The listing builds one solid part. Answer for the finished solid, in the listing's coordinates (mm). Face numbers are marked on the shaded views. A direction names the side the tool comes from. Round coordinates to 2 decimals unless told otherwise and drop trailing zeros. Write each loop counter-clockwise with the first axis right and the second up, starting at its lowest first coordinate (ties: lowest second). Pieces come first, ordered by that corner, then holes. Notation, with made-up numbers: M 32,-36.5 L 73,-36.5 A20 cw 73,2.5 Z; hole C -37,29 d1. An arc over 180 degrees is marked long. One line per item, written item: value. Start each with the question number.
(1) Given P1, Ø5, axis at x = -8.5, z = 8.5, coming from the +Y side; P2, Ø6, axis at x = 38, z = 12.5, coming from the -Y side; P3, Ø1.5, axis at y = 4.5, z = 11.5, coming from the +X side, each flat-ended and moving along its own axis, determine where each tip first touches the part or whether it passes through.
(2) For the marked faces 4 and 5, determine the directions among +Z, -Z, +X, -X, +Y, -Y from which every point of the face is accessible in a straight line to the end or side of a thin tool.
(3) Section D-D (x = 49.5) is taken. Determine the outline of the cut face in (y, z), plus the area to 3 significant figures.
(4) Consider probe 1 along Z at (x, y) = (-42.5, 13.5); probe 2 along Y at (x, z) = (0, 7) (3 decimals); probe 3 along X at (y, z) = (-3, 8). Determine where each line is inside the solid, lowest interval first.
(5) For a pull along Y with two mould halves and no side action, classify the marked faces 1, 2 and 3 as released by +Y, released by -Y, zero draft, split by the parting line, or undercut.
(6) Section A-A (x = 0) is taken. Determine the outline of the cut face in (y, z) (3 decimals).
(7) Section B-B (z = 7.5) is taken. State how many separate pieces and enclosed holes the cut face has, plus the area to 3 significant figures.
(8) Section C-C (x = -42.5) is taken. Determine the outline of the cut face in (y, z), plus the area to 4 significant figures.
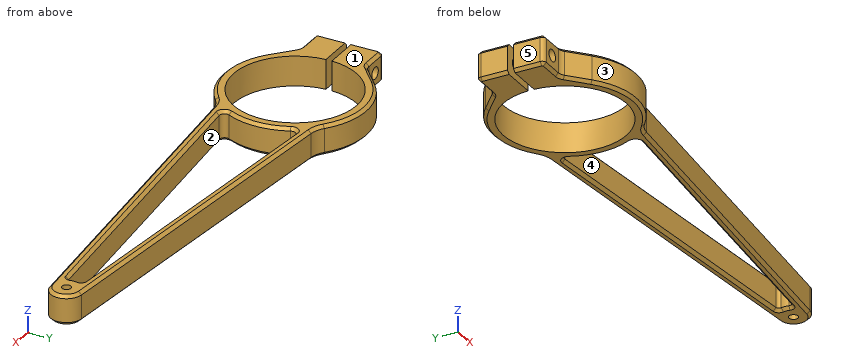
```python
from build123d import *

# Parameters (mm, degrees)
SKETCH_R     = 2.25
PAD_DEPTH    = 15
SKETCH001_R  = 3
HOLE_DEPTH   = 53.001
FILLET_R     = 5
FILLET001_R  = 2
FILLET002_R  = 12.5
FILLET003_R  = 2.5
FILLET004_R  = 1.5
CHAMFER_SIZE = 1.5


with BuildPart() as part:
    # Sketch → Pad (new body)
    with BuildSketch(Plane.XY):
        with BuildLine():
            ThreePointArc((-31.038776, -1.5), (31.075, 0), (-31.038776, 1.5))
            Line((-50, 1.5), (-31.038776, 1.5))
            Line((-50, 17), (-50, 1.5))
            Line((-35, 17), (-50, 17))
            Line((-35, 17), (-23.992027, 26.839945))
            ThreePointArc((25.903668, 25), (1.326628, 35.975548), (-23.992027, 26.839945))
            Line((25.903668, 25), (210.734184, 7.96624))
            ThreePointArc((210.734184, -7.96624), (218, 0), (210.734184, 7.96624))
            Line((25.903668, -25), (210.734184, -7.96624))
            ThreePointArc((-23.992027, -26.839945), (1.326628, -35.975548), (25.903668, -25))
            Line((-23.992027, -26.839945), (-35, -17))
            Line((-35, -17), (-50, -17))
            Line((-50, -1.5), (-50, -17))
            Line((-50, -1.5), (-31.038776, -1.5))
        make_face()
        with Locations((210, 0)):
            Circle(SKETCH_R, mode=Mode.SUBTRACT)
        with BuildLine():
            ThreePointArc((202.890406, 3.667925), (202, 0), (202.890406, -3.667925))
            Line((202.890406, -3.667925), (30.208298, -19.582102))
            ThreePointArc((30.208298, -19.582102), (36, 0), (30.208298, 19.582102))
            Line((30.208298, 19.582102), (202.890406, 3.667925))
        make_face(mode=Mode.SUBTRACT)
    extrude(amount=PAD_DEPTH)

    # Sketch001 (on Face13 of Pad) → Hole (cut, through all)
    with BuildSketch(Plane.XZ.offset(17)):
        with Locations((-42.5, 7.5)):
            Circle(SKETCH001_R)
    extrude(amount=-HOLE_DEPTH, mode=Mode.SUBTRACT)

    # Fillet
    fillet_edges = [part.edges().sort_by_distance(p)[0] for p in [
        (-35, -17, 7.5),
        (-35, 17, 7.5),
    ]]
    fillet(fillet_edges, radius=FILLET_R)

    # Fillet001
    fillet001_edges = [part.edges().sort_by_distance(p)[0] for p in [
        (-50, 17, 7.5),
        (-50, -17, 7.5),
    ]]
    fillet(fillet001_edges, radius=FILLET001_R)

    # Fillet002
    fillet002_edges = [part.edges().sort_by_distance(p)[0] for p in [
        (25.903668, -25, 7.5),
        (25.903668, 25, 7.5),
    ]]
    fillet(fillet002_edges, radius=FILLET002_R)

    # Fillet003
    fillet003_edges = [part.edges().sort_by_distance(p)[0] for p in [
        (30.208298, -19.582102, 7.5),
        (30.208298, 19.582102, 7.5),
    ]]
    fillet(fillet003_edges, radius=FILLET003_R)

    # Fillet004
    fillet004_edges = [part.edges().sort_by_distance(p)[0] for p in [
        (202.890406, 3.667925, 7.5),
        (202.890406, -3.667925, 7.5),
    ]]
    fillet(fillet004_edges, radius=FILLET004_R)

    # Chamfer
    chamfer_edges = [part.edges().sort_by_distance(p)[0] for p in [
        (120.438497, 16.287783, 15),
        (120.438497, 16.287783, 0),
        (117.936912, 11.497137, 15),
        (117.936912, 11.497137, 0),
    ]]
    chamfer(chamfer_edges, length=CHAMFER_SIZE)


solid = part.part
```
Recorded:
1. P1: stops at y = 35.5
1. P2: stops at y = -24.16
1. P3: stops at x = 217.07
2. face 4: +Z, -Z
2. face 5: +Z, -Z, -X, +Y, -Y
3. outline: M -22.83,1.5 L -21.32,0 L -19.31,0 L -17.8,1.5 L -17.8,13.5 L -19.31,15 L -21.32,15 L -22.83,13.5 Z; M 17.8,1.5 L 19.31,0 L 21.32,0 L 22.83,1.5 L 22.83,13.5 L 21.32,15 L 19.31,15 L 17.8,13.5 Z
3. area: 142 mm2
4. probe 1: z = 0 to 4.5, 10.5 to 15
4. probe 2: y = -36 to -31.075, 31.075 to 36
4. probe 3: x = -50 to -45.46, -39.54 to -30.93, 30.93 to 35.87, 202.15 to 217.42
5. face 1: zero draft
5. face 2: undercut
5. face 3: released by -Y
6. outline: M -36,1.5 L -34.5,0 L -31.075,0 L -31.075,15 L -34.5,15 L -36,13.5 Z; M 31.075,0 L 34.5,0 L 36,1.5 L 36,13.5 L 34.5,15 L 31.075,15 Z
7. separate pieces: 3
7. enclosed holes: 2
7. area: 3,320 mm2
8. outline: M -17,1.5 L -15.5,0 L -1.5,0 L -1.5,4.5 L -17,4.5 Z; M -17,10.5 L -1.5,10.5 L -1.5,15 L -15.5,15 L -17,13.5 Z; M 1.5,0 L 15.5,0 L 17,1.5 L 17,4.5 L 1.5,4.5 Z; M 1.5,10.5 L 17,10.5 L 17,13.5 L 15.5,15 L 1.5,15 Z
8. area: 274.5 mm2
